```python
from build123d import *

# Parameters (mm, degrees)
SKETCH1_R               = 18
BOSS_EXTRUDE1_DEPTH     = 24
CUT_EXTRUDE1_DEPTH      = 24
CUT_EXTRUDE1_DEPTH_BACK = 24
SKETCH2_R               = 8
DOME1_FACE_RADIUS       = 18
DOME1_HEIGHT            = 4
SKETCH5_R               = 12
BOSS_EXTRUDE3_DEPTH     = 208
SKETCH13_R              = 10
BOSS_EXTRUDE4_DEPTH     = 20
M8_TAPPED_HOLE1_D       = 6.8
M8_TAPPED_HOLE1_DEPTH   = 20
M8_TAPPED_HOLE1_TIP     = 2.042926105


with BuildPart() as part:
    # Sketch1 → Boss-Extrude1 (new body)
    with BuildSketch(Plane(origin=(0, 0, 0), x_dir=(1, 0, 0), z_dir=(0, 1, 0))):
        with Locations(Location((0, 0, 0), (0, 0, 270))):
            Circle(SKETCH1_R)
    extrude(amount=BOSS_EXTRUDE1_DEPTH)

    # Sketch2 → Cut-Extrude1 (cut, two sides: drawn at the far end of the back side and taken through both)
    with BuildSketch(Plane(origin=(0, 0, 0), x_dir=(0, 0, -1), z_dir=(1, 0, 0)).offset(-CUT_EXTRUDE1_DEPTH_BACK)):
        with Locations(Location((0, 12, 0), (0, 0, 180))):
            Circle(SKETCH2_R)
    extrude(amount=CUT_EXTRUDE1_DEPTH + CUT_EXTRUDE1_DEPTH_BACK, mode=Mode.SUBTRACT)

    # Dome1: a dome of height H over a round flat face of radius A is a cap of a sphere of radius (A * A + H * H) / (2 * H)
    dome1_r = (DOME1_FACE_RADIUS * DOME1_FACE_RADIUS + DOME1_HEIGHT * DOME1_HEIGHT) / (2 * DOME1_HEIGHT)
    dome1_base = Plane((0, 24, 0), z_dir=(0, 1, 0))
    with Locations(dome1_base.offset(DOME1_HEIGHT - dome1_r)):
        dome1_ball = Sphere(dome1_r, mode=Mode.PRIVATE)
    add(split(dome1_ball, bisect_by=dome1_base, keep=Keep.TOP, mode=Mode.PRIVATE))

    # Sketch3 → Revolve1 (revolve)
    with BuildSketch(Plane(origin=(0, 0, 0), x_dir=(0, 0, -1), z_dir=(1, 0, 0)), mode=Mode.PRIVATE) as revolve1_sk:
        Polygon((0, 0), (0, -2.828427125), (15.171572875, -2.828427125), (18, 0), align=None)
    revolve(revolve1_sk.sketch.rotate(Axis((0, 0, 0), (0, -1, 0)), 180), axis=Axis((0, 0, 0), (0, -1, 0)))

    # Sketch5 → Boss-Extrude3 (add)
    with BuildSketch(Plane(origin=(0, 0, 0), x_dir=(1, 0, 0), z_dir=(0, 1, 0))):
        with Locations(Location((0, 0, 0), (0, 0, 270))):
            Circle(SKETCH5_R)
    extrude(amount=-BOSS_EXTRUDE3_DEPTH)

    # Sketch13 → Boss-Extrude4 (add)
    with BuildSketch(Plane(origin=(0, -208, 0), x_dir=(-1, 0, 0), z_dir=(0, -1, 0))):
        with Locations(Location((0, 0, 0), (0, 0, 270))):
            Circle(SKETCH13_R)
    extrude(amount=BOSS_EXTRUDE4_DEPTH)

    # Sketch14 → Revolve2 (revolve)
    with BuildSketch(Plane(origin=(0, 0, 0), x_dir=(0, 0, -1), z_dir=(1, 0, 0))):
        Polygon((0, -228), (0, -230), (-8, -230), (-10, -228), align=None)
    revolve(axis=Axis((0, -228, 0), (0, -1, 0)))

    # M8 Tapped Hole1
    with Locations(Plane(origin=(0, -230, 0), x_dir=(-1, 0, 0), z_dir=(0, -1, 0))):
        with Locations((0, 0)):
            Hole(M8_TAPPED_HOLE1_D / 2, depth=M8_TAPPED_HOLE1_DEPTH)
            with Locations((0, 0, -(M8_TAPPED_HOLE1_DEPTH + M8_TAPPED_HOLE1_TIP / 2))):  # 118° drill point
                Cone(0, M8_TAPPED_HOLE1_D / 2, M8_TAPPED_HOLE1_TIP, mode=Mode.SUBTRACT)


solid = part.part
```
Build history of the part. All positions in model axes, mm. A direction names the side the tool comes from. Coordinates: 2 decimals unless noted, no trailing zeros. Order: outer loops, then holes, each group sorted by start corner. A loop starts at its lowest first (then second) coordinate and runs counter-clockwise, first axis right, second up.
Item 1: Drill centre lines: L1, parallel to Z at x = -0.5, y = -183; L2, parallel to X at y = -198, z = 1; L3, parallel to Y at x = 2.5, z = 0. Where is each one in solid material? Low to high.
Filled in:
L1: z = -11.99 to 11.99
L2: x = -11.96 to 11.96
L3: y = -209.46 to 4, 20 to 27.93
Item 2: Drop flat-ended pins along their axis: pin 1 Ø11 at (x, z) = (0, 0) entering from -Y; pin 2 Ø10 at (x, y) = (13, -119.5) entering from +Z; pin 3 Ø1 at (x, z) = (1.5, 4.5) entering from +Y; pin 4 Ø3 at (x, z) = (-10.5, -0.5) entering from -Y. Give the stop position or say it passes through.
Filled in:
pin 1: stops at y = -230
pin 2: stops at z = 8.94
pin 3: stops at y = 27.79
pin 4: stops at y = -228.99
Item 3: Tool access for faces 1 (the cylindrical face through (5.407, 11.832, 17.169)), 2 (the cylindrical face through (9.76, -217.86, -2.17)): list every direction of +Z, -Z, +X, -X, +Y, -Y with a clear straight run to the whole face (end or side of a thin tool).
Filled in:
face 1: +Y, -Y
face 2: -Y
Item 4: Mould opens along Z. For faces 3 (the flat face through (9, -208, -5)), 4 (the cylindrical face through (3.604, -103.978, 11.446)), 5 (the conical face through (0.128, -208.312, 0.576)) say: released by +Z, released by -Z, zero draft, split by the parting line, or undercut.
Filled in:
face 3: zero draft
face 4: split by the parting line
face 5: undercut
Item 5: Saw through at A-A on y = -204.5. List the corners of the cut face in (x, z), then the cut area to 3 significant figures.
Filled in:
outline: circle Ø24 at (0, 0)
area: 452 mm2
Item 6: Saw through at B-B on y = 12. List the corners of the cut face in (x, z), then the cut area to 3 significant figures.
Filled in:
outline: (-16.12, -8) arc R18 ccw to (16.12, -8) - close; (-16.12, 8) - (16.12, 8) arc R18 ccw to start
area: 461 mm2
